from build123d import *

# Parameters (mm, degrees)
SKETCH1_W           = 125
SKETCH1_H           = 75
BOSS_EXTRUDE1_DEPTH = 15
SKETCH2_W           = 35
SKETCH2_H           = 46
CUT_EXTRUDE4_DEPTH  = 5
SKETCH3_W           = 5.6
SKETCH3_H           = 30
CUT_EXTRUDE5_DEPTH  = 5


with BuildPart() as part:
    # Sketch1 → Boss-Extrude1 (new body)
    with BuildSketch(Plane(origin=(0, 0, 0), x_dir=(1, 0, 0), z_dir=(0, 1, 0))):
        with Locations((62.5, 37.5)):
            Rectangle(SKETCH1_W, SKETCH1_H)
    extrude(amount=BOSS_EXTRUDE1_DEPTH)

    # Sketch2 → Cut-Extrude4 (cut)
    with BuildSketch(Plane(origin=(0, 15, 0), x_dir=(1, 0, 0), z_dir=(0, 1, 0))):
        Polygon((53.5, 64.5), (125, 64.5), (125, 49.5), (123, 49.5), (123, 35.5), (125, 35.5), (125, 15.5), (123, 15.5), (123, 10.5), (53.5, 10.5), align=None)
        with Locations((26, 37.5)):
            Rectangle(SKETCH2_W, SKETCH2_H)
    extrude(amount=-CUT_EXTRUDE4_DEPTH, mode=Mode.SUBTRACT)

    # Sketch3 → Cut-Extrude5 (cut)
    with BuildSketch(Plane.XZ):
        with Locations((17.8, -37.5)):
            Rectangle(SKETCH3_W, SKETCH3_H)
        with Locations((107.2, -37.5)):
            Rectangle(SKETCH3_W, SKETCH3_H)
    extrude(amount=-CUT_EXTRUDE5_DEPTH, mode=Mode.SUBTRACT)


solid = part.part
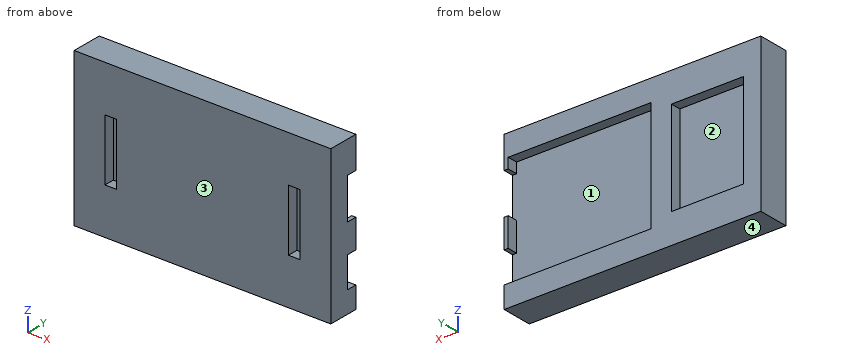
For this review, take the finished solid that the model builds, in its own axes (mm). Face numbers are marked on the shaded views. Round coordinates to 2 decimals unless told otherwise and drop trailing zeros. Order: outer loops, then holes, each group sorted by start corner. A loop starts at its lowest first (then second) coordinate and runs counter-clockwise, first axis right, second up. Notation, with made-up numbers: (64, -27) -> (88, -27) arc R15 cw to (88, -8) -> close; hole circle Ø4 at (61, 80). An arc over 180 degrees is marked (long way). Write item = value, one per line. Start each with the question number.
1) Take a section at C-C on z = -32. State the section outline as (x, y) points.
2) Take a section at B-B on x = 11. State the section outline as (y, z) points.
3) To check wall thickness, follow line 1 (X direction, y = 1.5, z = -31); line 2 (X direction, y = 14.5, z = -13); line 3 (X direction, y = 13.25, z = -46.5). State the ranges of each line that lie inside material, in increasing order. Write a range as from..to.
4) The part is to be moulded in two halves that separate along Z. For the marked faces 1, 2, 3 and 4, say which applies: +Z half, -Z half, draft (parallel to the pull), parting line (faces both ways), or undercut.
5) Take a section at D-D on y = 3.25. State the section outline as (x, z) points, plus the area to 3 significant figures.
6) Take a section at A-A on y = 12. State the section outline as (x, z) points, plus the area to 3 significant figures.
7) Insertion check: pin 1 (1 mm diameter, centred on x = 36.5, z = -32, fed in from +Y); pin 2 (1.7 mm diameter, centred on x = 16.5, z = -39, fed in from -Y). Each pin has a flat end and moves straight along its axis. Give the tip position at first contact, or say it passes through.
Verdict:
q1.outline = (0, 0) -> (15, 0) -> (15, 5) -> (20.6, 5) -> (20.6, 0) -> (104.4, 0) -> (104.4, 5) -> (110, 5) -> (110, 0) -> (125, 0) -> (125, 10) -> (53.5, 10) -> (53.5, 15) -> (43.5, 15) -> (43.5, 10) -> (8.5, 10) -> (8.5, 15) -> (0, 15) -> close
q2.outline = (0, -75) -> (15, -75) -> (15, -60.5) -> (10, -60.5) -> (10, -14.5) -> (15, -14.5) -> (15, 0) -> (0, 0) -> close
q3.line_1 = 0..15, 20.6..104.4, 110..125
q3.line_2 = 0..53.5, 123..125
q3.line_3 = 0..8.5, 43.5..53.5, 123..125
q4.face_1 = undercut
q4.face_2 = undercut
q4.face_3 = draft
q4.face_4 = -Z half
q5.outline = (0, -75) -> (125, -75) -> (125, 0) -> (0, 0) -> close; hole (15, -52.5) -> (20.6, -52.5) -> (20.6, -22.5) -> (15, -22.5) -> close; hole (104.4, -52.5) -> (110, -52.5) -> (110, -22.5) -> (104.4, -22.5) -> close
q5.area = 9,040 mm2
q6.outline = (0, -75) -> (125, -75) -> (125, -64.5) -> (53.5, -64.5) -> (53.5, -10.5) -> (123, -10.5) -> (123, -15.5) -> (125, -15.5) -> (125, 0) -> (0, 0) -> close; (123, -49.5) -> (125, -49.5) -> (125, -35.5) -> (123, -35.5) -> close; hole (8.5, -60.5) -> (43.5, -60.5) -> (43.5, -14.5) -> (8.5, -14.5) -> close
q6.area = 3,940 mm2
q7.pin_1 = 10
q7.pin_2 = 5
